Check sheet for the modelled part. Datum: model origin and axes. Units: mm. Round coordinates to 2 decimals unless told otherwise and drop trailing zeros. Loops run counter-clockwise (first coordinate to the right, second up) from the corner with the lowest first, then second, coordinate; pieces in that order, holes last. Notation, with made-up numbers: (5.25, 27) - (27.25, 27) arc R23 ccw to (27.25, 50) - close; hole circle Ø9 at (63, 14.25). An arc over 180 degrees is marked (long way). Return JSON: item names as keys, results as strings.
from build123d import *

# Parameters (mm, degrees)
NRG_PSU_CASE_1_START = -230.550293706
NRG_PSU_CASE_1_DEPTH = 165.1
SKETCH2_W            = 10.16
SKETCH2_H            = 30.52357951
CUT_EXTRUDE1_DEPTH   = 1.27
FILLET1_R            = 15.24


# Read off the part's stored shape, not the designer's step: -NRG_PSU_CASE-1
with BuildPart() as part:
    # -NRG_PSU_CASE-1 outline → -NRG_PSU_CASE-1 (new body)
    with BuildSketch(Plane.YZ.offset(NRG_PSU_CASE_1_START)):
        Polygon((42.926, 50.844880664), (36.249795103, 57.521085561), (36.249795103, -47.060903743), (42.926, -40.384698846), align=None)
    extrude(amount=NRG_PSU_CASE_1_DEPTH)

    # Sketch2 → Cut-Extrude1 (cut)
    with BuildSketch(Plane(origin=(0, 42.926, 0), x_dir=(1, 0, 0), z_dir=(0, 1, 0))):
        with Locations((-215.310293706, -5.230090909)):
            Rectangle(SKETCH2_W, SKETCH2_H)
    extrude(amount=-CUT_EXTRUDE1_DEPTH, mode=Mode.SUBTRACT)

    # Fillet1
    # the kernel refuses this fillet: 15.24 mm, written as the material it adds along each edge
    with BuildSketch(Plane(origin=(-195.00352862, 41.656, 20.491880664), x_dir=(0, 1, 0), z_dir=(-1, 0, 0)), Plane(origin=(-220.390293706, 41.656, -10.031698846), x_dir=(0, 1, 0), z_dir=(1, 0, 0))) as fillet1_piece_1:
        with BuildLine():
            CenterArc((15.24, 6.090706035), FILLET1_R, 180, 23.556464309)
            Line((0, 6.090706035), (0, 0))
            Line((0, 0), (1.27, 0))
        make_face()
    extrude(amount=25.386765087)


solid = part.part
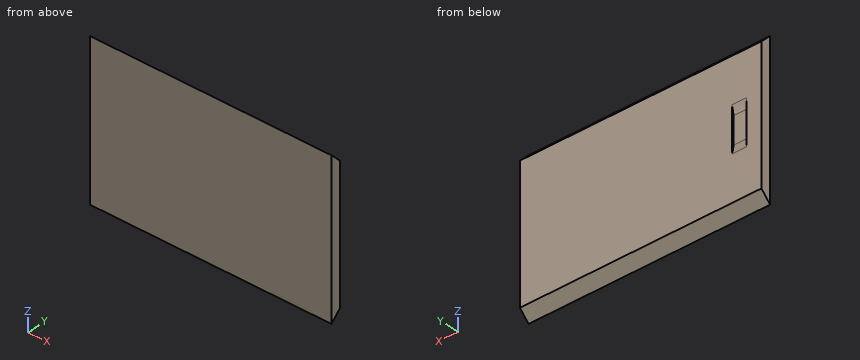
Q1. Sectioned sample at A-A (x = -193). Enter the section's corners in (y, z).
Answer key:
{"outline": "(36.25, -47.06) - (42.93, -40.38) - (42.93, 50.84) - (36.25, 57.52) - close"}
Q2. Depth check by flat-ended pin: P1, Ø3, axis at x = -154, y = 37.5, coming from the -Z side; P2, Ø8, axis at x = -215, z = 8.5, coming from the +Y side; P3, Ø2, axis at x = -130.5, y = 39.5, coming from the -Z side. Enter the tip coordinate at first touch or a pass-through.
Answer key:
{"P1": "stops at z = -47.06", "P2": "stops at y = 41.66", "P3": "stops at z = -44.81"}
Q3. Sectioned sample at B-B (y = 39.75). Enter the section's corners in (x, z).
Answer key:
{"outline": "(-230.55, -43.56) - (-65.45, -43.56) - (-65.45, 54.02) - (-230.55, 54.02) - close"}
Q4. Scan lines: probe 1 along X at (y, z) = (42.5, 15); probe 2 along Z at (x, y) = (-83, 40.5); probe 3 along Z at (x, y) = (-166, 39.5). Record each from-to range of solid material in increasing order. Write a range as [from, to].
Answer key:
{"probe 1": "x = [-230.55, -220.39], [-210.23, -65.45]", "probe 2": "z = [-42.81, 53.27]", "probe 3": "z = [-43.81, 54.27]"}
